from build123d import *

# Parameters (mm, degrees)
BOSS_EXTRUDE1_DEPTH = 1
BOSS_EXTRUDE2_DEPTH = 12.58
SKETCH1_4_W         = 149.48
SKETCH1_4_H         = 2
BOSS_EXTRUDE3_DEPTH = 15.58
SKETCH1_5_W         = 92.02
SKETCH1_5_H         = 2
BOSS_EXTRUDE4_DEPTH = 1


with BuildPart() as part:
    # Sketch1 → Boss-Extrude1 (new body)
    with BuildSketch(Plane(origin=(0, 0, 0), x_dir=(1, 0, 0), z_dir=(0, 1, 0))):
        Polygon((-50.01, 19.39179677), (-101.494739838, 19.39179677), (-112.690598923, 0), (-109.845299462, -4.92820323), (-74.74, -4.92820323), (74.74, -4.92820323), (109.845299462, -4.92820323), (112.690598923, 0), (101.494739838, 19.39179677), (42.01, 19.39179677), align=None)
    extrude(amount=BOSS_EXTRUDE1_DEPTH)

    # Sketch1<3> → Boss-Extrude2 (add)
    with BuildSketch(Plane(origin=(0, 0, 0), x_dir=(1, 0, 0), z_dir=(0, 1, 0))):
        Polygon((-115, 0), (-111, -6.92820323), (-74.74, -6.92820323), (-74.74, -4.92820323), (-109.845299462, -4.92820323), (-112.690598923, 0), (-101.494739838, 19.39179677), (-102.649440377, 21.39179677), align=None)
        Polygon((115, 0), (111, -6.92820323), (74.74, -6.92820323), (74.74, -4.92820323), (109.845299462, -4.92820323), (112.690598923, 0), (101.494739838, 19.39179677), (102.649440377, 21.39179677), align=None)
    extrude(amount=BOSS_EXTRUDE2_DEPTH)

    # Sketch1<4> → Boss-Extrude3 (add)
    with BuildSketch(Plane(origin=(0, 0, 0), x_dir=(1, 0, 0), z_dir=(0, 1, 0))):
        Polygon((-102.649440377, 21.39179677), (-101.494739838, 19.39179677), (-50.01, 19.39179677), (-50.01, 21.39179677), align=None)
        Polygon((102.649440377, 21.39179677), (101.494739838, 19.39179677), (42.01, 19.39179677), (42.01, 21.39179677), align=None)
        with Locations((0, -5.92820323)):
            Rectangle(SKETCH1_4_W, SKETCH1_4_H)
    extrude(amount=BOSS_EXTRUDE3_DEPTH)

    # Sketch1<5> → Boss-Extrude4 (add)
    with BuildSketch(Plane(origin=(0, 0, 0), x_dir=(1, 0, 0), z_dir=(0, 1, 0))):
        with Locations((-4, 20.39179677)):
            Rectangle(SKETCH1_5_W, SKETCH1_5_H)
    extrude(amount=BOSS_EXTRUDE4_DEPTH)


solid = part.part
Could you check a few things on this model? Use its own coordinates, in mm. A direction names the side the tool comes from. Give positions to 0.01 mm unless a question says otherwise; leave off trailing zeros. Order: outer loops, then holes, each group sorted by start corner. A loop starts at its lowest first (then second) coordinate and runs counter-clockwise, first axis right, second up.
1. Suppose I cut it at A-A (y = 6.5). Write out the boundary of the cut face in (x, z), plus the area to 3 significant figures.
Answers below:
outline: (-115, 0) - (-102.65, -21.39) - (-50.01, -21.39) - (-50.01, -19.39) - (-101.49, -19.39) - (-112.69, 0) - (-109.85, 4.93) - (109.85, 4.93) - (112.69, 0) - (101.49, -19.39) - (42.01, -19.39) - (42.01, -21.39) - (102.65, -21.39) - (115, 0) - (111, 6.93) - (-111, 6.93) - close
area: 788 mm2
2. I need wall thicknesses on L1, parallel to Z at x = -73, y = 10; L2, parallel to Z at x = -8, y = 12; L3, parallel to Y at x = -60.5, z = -17. Which ranges of each line are inside material? Lowest first, please.
Answers below:
L1: z = -21.39 to -19.39, 4.93 to 6.93
L2: z = 4.93 to 6.93
L3: y = 0 to 1
3. For pin 1 (14 mm diameter, centred on x = 98, z = -9, fed in from +Y); pin 2 (1.6 mm diameter, centred on y = 13.5, z = 6, fed in from +X); pin 3 (1 mm diameter, centred on y = 13.5, z = 6, fed in from -X), each with a flat end and sliding along its axis, tell me the tip position at first contact or that it passes through.
Answers below:
pin 1: stops at y = 1
pin 2: stops at x = 74.74
pin 3: stops at x = -74.74
4. Suppose I cut it at B-B (x = -72). Write out the boundary of the cut face in (y, z), plus the area to 3 significant figures.
Answers below:
outline: (0, -21.39) - (15.58, -21.39) - (15.58, -19.39) - (1, -19.39) - (1, 4.93) - (15.58, 4.93) - (15.58, 6.93) - (0, 6.93) - close
area: 86.6 mm2
5. Thinking about a two-plate mould opening in Z: for faces 1 (the flat face through (-2, 1, -8)), 2 (the flat face through (-99.4, 12.58, 5.3)), 3 (the flat face through (111.248, 6.709, 2.499)), 4 (the flat face through (-1.4, 0.8, -21.392)), which applies, +Z half, -Z half, draft (parallel to the pull), parting line (faces both ways), or undercut?
Answers below:
face 1: undercut
face 2: draft
face 3: undercut
face 4: -Z half
6. Which directions (+Z, -Z, +X, -X, +Y, -Y) give clear straight access to the entire face, cutting with the end or side of a thin tool? Please do faces 5 (the flat face through (107.17, 6.71, -9.56)), 6 (the flat face through (-2, 8, 6.928)), 7 (the flat face through (99.4, 12.58, 5.3)).
Answers below:
face 5: +Y
face 6: +Z, +X, -X, +Y, -Y
face 7: +Z, +X, +Y
7. Suppose I cut it at C-C (z = -16). Write out the boundary of the cut face in (x, y).
Answers below:
outline: (-105.76, 0) - (105.76, 0) - (105.76, 12.58) - (103.45, 12.58) - (103.45, 1) - (-103.45, 1) - (-103.45, 12.58) - (-105.76, 12.58) - close
8. Suppose I cut it at D-D (x = -35). Write out the boundary of the cut face in (y, z).
Answers below:
outline: (0, -21.39) - (1, -21.39) - (1, 4.93) - (15.58, 4.93) - (15.58, 6.93) - (0, 6.93) - close
